Answer from the drawing. Dimensions are ordinates in mm from the lowest x, y and z of the part. Give positions to 0.01 mm unless a question says otherwise; leave off trailing zeros. Write each loop counter-clockwise with the first axis right and the second up, starting at its lowest first coordinate (ties: lowest second). Pieces come first, ordered by that corner, then holes. Notation, with made-up numbers: (66.25, -33.5) - (95.25, -33.5) arc R28 ccw to (95.25, -6.5) - close; hole circle Ø6 at (28, 11). An arc over 180 degrees is marked (long way). Answer as a JSON object with one key per item and string values. Group by question number.
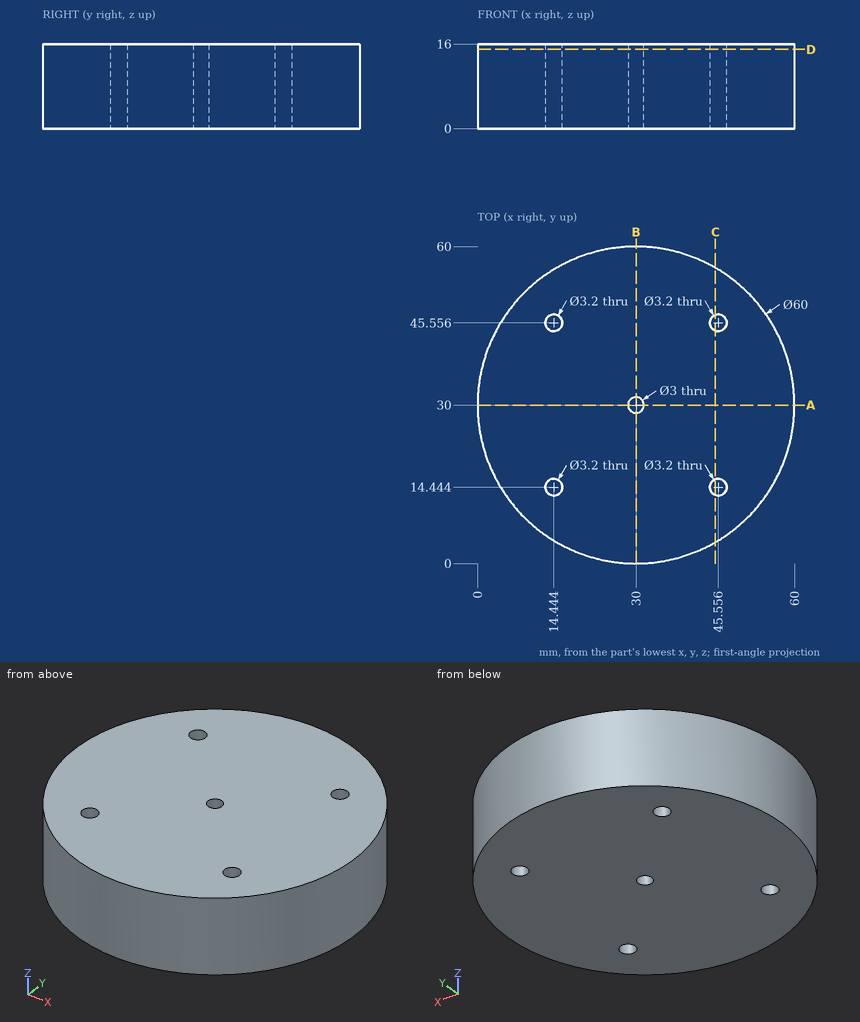
1) Find section C-C, the plane x = 45. Write down the section's boundary in (y, z).
2) Find the intervals of material crossed by line 1 (X direction, y = 14.5, z = 11.25) (1 decimal); line 2 (Y direction, x = 29, z = 13.5) (1 decimal); line 3 (X direction, y = 47, z = 11.75) (1 decimal), in increasing order. Write a range as [from, to].
3) Find section A-A, the plane y = 30. Write down the section's boundary in (x, z), and give its area (3 significant figures).
4) Flat-ended cylindrical pins translate along their axes: pin 1 Ø8 at (x, z) = (46.5, 13.5) entering from -Y; pin 2 Ø8 at (y, z) = (13, 12) entering from +X; pin 3 Ø3 at (y, z) = (42, 5.5) entering from -X. Find the tip coordinate at first contact, or state that the pin passes through.
5) Find section D-D, the plane z = 15. Write down the section's boundary in (x, y), and give its area (3 significant figures).
Values follow:
{
 "1": {"outline": "(4.02, 0) - (12.94, 0) - (12.94, 16) - (4.02, 16) - close; (15.94, 0) - (44.06, 0) - (44.06, 16) - (15.94, 16) - close; (47.06, 0) - (55.98, 0) - (55.98, 16) - (47.06, 16) - close"},
 "2": {"line 1": "x = [4.3, 12.8], [16, 44], [47.2, 55.7]", "line 2": "y = [0, 28.9], [31.1, 60]", "line 3": "x = [5.3, 13.8], [15.1, 44.9], [46.2, 54.7]"},
 "3": {"outline": "(0, 0) - (28.5, 0) - (28.5, 16) - (0, 16) - close; (31.5, 0) - (60, 0) - (60, 16) - (31.5, 16) - close", "area": "912 mm2"},
 "4": {"pin 1": "stops at y = 2.73", "pin 2": "stops at x = 57.04", "pin 3": "stops at x = 1.9"},
 "5": {"outline": "circle Ø60 at (30, 30); hole circle Ø3.2 at (14.44, 14.44); hole circle Ø3.2 at (14.44, 45.56); hole circle Ø3 at (30, 30); hole circle Ø3.2 at (45.56, 14.44); hole circle Ø3.2 at (45.56, 45.56)", "area": "2,790 mm2"}
}
